Can you work these out from the model? Positions are in its coordinate system, mm. A direction names the side the tool comes from. Coordinates: 2 decimals unless noted, no trailing zeros. Order: outer loops, then holes, each group sorted by start corner. A loop starts at its lowest first (then second) coordinate and runs counter-clockwise, first axis right, second up. Notation, with made-up numbers: (-9, 83) - (-4, 83) arc R10 cw to (-4, 90) - close; hole circle Ø6 at (15.25, 35.5). An arc over 180 degrees is marked (long way). Return JSON: item names as keys, results as strings. Group by question number.
1) If I drill on line 1 along Z through (x, y) = (-95, 39.5); line 2 along X through (y, z) = (69.5, 89); line 3 along X through (y, z) = (42, 19), over which ranges is the centre line in solid material (lowest first)?
2) Imagine slicing it at B-B (x = -91.5). Write out the boundary of the cut face in (y, z).
3) Imagine slicing it at D-D (z = 70). Write out the boundary of the cut face in (x, y), and give its area (3 significant figures).
4) Imagine slicing it at C-C (y = 32). Write out the boundary of the cut face in (x, z), and give its area (3 significant figures).
5) Imagine slicing it at A-A (y = 64). Write out the boundary of the cut face in (x, z).
6) If we mould it in two halves opening along Z, with no side actions, what happens to faces 6 (the face through (-76, 11, 105.259)), 7 (the face through (38.401, 31, 52)), 8 (the face through (-75, 72, 68.159))? For each: pulls with the +Z half, pulls with the -Z half, needs draft (parallel to the pull), parting line crosses it, or undercut.
7) Which directions (+Z, -Z, +X, -X, +Y, -Y) give clear straight access to the entire face, cutting with the end or side of a thin tool? Please do faces 1 (the face through (-38, 82.151, 52)), 2 (the face through (-111.599, 31, 52)), 3 (the face through (-42.439, 11, 93)), 4 (the face through (-75, 77.151, 73)), 5 (the face through (-38, 32, 79.502)).
8) For pin 1 Ø2 at (x, y) = (-86, 36.5) entering from +Z; pin 2 Ø7 at (x, z) = (-90, 74) entering from -Y; pin 3 Ø1.5 at (x, y) = (13, 69.5) entering from +Z, each with a flat end and sliding along its axis, tell me the tip position at first contact or that it passes through.
```python
from build123d import *

# Parameters (mm, degrees)
F0_W      = 150
F0_H      = 100
F1_DEPTH  = 5
F2_W      = 5
F2_H      = 100
F3_DEPTH  = 100
F4_W      = 145
F4_H      = 5
F5_DEPTH  = 100
F6_W      = 5
F6_H      = 95
F7_DEPTH  = 100
F8_W      = 140
F8_H      = 5
F9_DEPTH  = 100
F10_W     = 140
F10_H     = 5
F11_DEPTH = 36.8
F12_W     = 10.8797177672
F12_H     = 90
F13_DEPTH = 36.8
F15_W     = 64.1449913383
F15_H     = 8.8397674263
F16_DEPTH = 36.8
F17_W     = 9.7464099526
F17_H     = 48.5053984448
F18_DEPTH = 37.1
F19_DEPTH = 1
F20_W     = 139.6295134723
F20_H     = 18.2434022427
F21_DEPTH = 85
F22_W     = 95
F22_H     = 2.5124400854
F23_DEPTH = 142.2
F25_DEPTH = 3


with BuildPart() as f1:
    # F0 (on Top) → F1 (new body)
    with BuildSketch(Plane.XY):
        with Locations((-36.598560214, 32.1514412761)):
            Rectangle(F0_W, F0_H)
    extrude(amount=F1_DEPTH)

    # F2 (on face) → F3 (join)
    with BuildSketch(Plane.XY.offset(5)):
        with Locations((-109.098560214, 32.1514412761)):
            Rectangle(F2_W, F2_H)
    extrude(amount=F3_DEPTH)

    # F4 (on face) → F5 (join)
    with BuildSketch(Plane.XY.offset(5)):
        with Locations((-34.098560214, 79.6514412761)):
            Rectangle(F4_W, F4_H)
    extrude(amount=F5_DEPTH)

    # F6 (on face) → F7 (join)
    with BuildSketch(Plane.XY.offset(5)):
        with Locations((35.901439786, 29.6514412761)):
            Rectangle(F6_W, F6_H)
    extrude(amount=F7_DEPTH)

    # F8 (on face) → F9 (join)
    with BuildSketch(Plane.XZ.offset(17.8485587239)):
        with Locations((-36.598560214, 65.6586462259)):
            Rectangle(F8_W, F8_H)
    extrude(amount=-F9_DEPTH)

    # F10 (on face) → F11 (join)
    with BuildSketch(Plane.XY.offset(68.1586462259)):
        with Locations((-36.598560214, -15.3485587239)):
            Rectangle(F10_W, F10_H)
    extrude(amount=F11_DEPTH)

    # F12 (on face) → F13 (join)
    with BuildSketch(Plane.XY.offset(68.1586462259)):
        with Locations((-36.9987897575, 32.1514412761)):
            Rectangle(F12_W, F12_H)
    extrude(amount=F13_DEPTH)

    # F15 (on face) → F16 (join)
    with BuildSketch(Plane.XY.offset(68.1586462259)):
        with Locations((-74.5111443102, 40.5214224011)):
            Rectangle(F15_W, F15_H)
    extrude(amount=F16_DEPTH)

    # F17 (on face) → F18 (join)
    with BuildSketch(Plane.XY.offset(68.1586462259)):
        with Locations((-75.8711062372, 11.1688547768)):
            Rectangle(F17_W, F17_H)
    extrude(amount=F18_DEPTH)

    # F19 (add): a face of the model
    f19_faces = [f1.faces().sort_by_distance(p)[0] for p in [
        (-75.8711062372, 35.4215539992, 86.7086462259),
    ]]
    extrude(f19_faces, amount=F19_DEPTH)

    # F20 (on face) → F21 (cut)
    with BuildSketch(Plane.XZ.offset(17.8485587239)):
        with Locations((-36.7838034779, 72.2803473473)):
            Rectangle(F20_W, F20_H)
    extrude(amount=-F21_DEPTH, mode=Mode.SUBTRACT)

    # F22 (on face) → F23 (join)
    with BuildSketch(Plane.YZ.offset(-106.598560214)):
        with Locations((29.6514412761, 78.2460346818)):
            Rectangle(F22_W, F22_H)
    extrude(amount=F23_DEPTH)

    # F24 (on face) → F25 (join)
    with BuildSketch(Plane(origin=(0, 0, 81.4020484686), x_dir=(1, 0, 0), z_dir=(0, 0, -1))):
        Polygon((33.0309532583, 17.8485587239), (-106.598560214, 17.8485587239), (-106.598560214, 12.8485587239), (-80.7443112135, 12.8485587239), (-70.9979012609, 12.8485587239), (-42.4386486411, 12.8485587239), (-31.5589308739, 12.8485587239), (33.0309532583, 12.8485587239), align=None)
    extrude(amount=F25_DEPTH)


solid = f1.part
```
Calculated:
{
 "1": {"line 1": "0 to 5, 76.99 to 79.5, 81.4 to 104.96", "line 2": "-111.6 to -106.6, -42.44 to -31.56, 33.4 to 38.4", "line 3": "-111.6 to -106.6, 33.4 to 38.4"},
 "2": {"outline": "(-17.85, 0) - (82.15, 0) - (82.15, 105) - (77.15, 105) - (77.15, 79.5) - (-12.85, 79.5) - (-12.85, 104.96) - (-17.85, 104.96) - (-17.85, 76.99) - (77.15, 76.99) - (77.15, 68.16) - (67.15, 68.16) - (67.15, 63.16) - (77.15, 63.16) - (77.15, 5) - (-17.85, 5) - close; (36.1, 81.4) - (44.94, 81.4) - (44.94, 104.96) - (36.1, 104.96) - close"},
 "3": {"outline": "(-111.6, -17.85) - (-106.6, -17.85) - (-106.6, 77.15) - (-42.44, 77.15) - (-42.44, 67.15) - (-31.56, 67.15) - (-31.56, 77.15) - (33.4, 77.15) - (33.4, -12.85) - (33.03, -12.85) - (33.03, -17.85) - (38.4, -17.85) - (38.4, 82.15) - (-111.6, 82.15) - close", "area": "1,810 mm2"},
 "4": {"outline": "(-111.6, 0) - (38.4, 0) - (38.4, 105) - (33.4, 105) - (33.4, 79.5) - (-106.6, 79.5) - (-106.6, 105) - (-111.6, 105) - close; (-80.74, 81.4) - (-71, 81.4) - (-71, 105.26) - (-80.74, 105.26) - close; (-42.44, 81.4) - (-31.56, 81.4) - (-31.56, 104.96) - (-42.44, 104.96) - close; hole (-106.6, 5) - (33.4, 5) - (33.4, 63.16) - (33.03, 63.16) - (33.03, 68.16) - (33.4, 68.16) - (33.4, 76.99) - (-106.6, 76.99) - close", "area": "2,590 mm2"},
 "5": {"outline": "(-111.6, 0) - (38.4, 0) - (38.4, 105) - (33.4, 105) - (33.4, 79.5) - (-106.6, 79.5) - (-106.6, 105) - (-111.6, 105) - close; (-42.44, 81.4) - (-31.56, 81.4) - (-31.56, 104.96) - (-42.44, 104.96) - close; hole (-106.6, 5) - (33.4, 5) - (33.4, 63.16) - (33.03, 63.16) - (33.03, 68.16) - (33.4, 68.16) - (33.4, 76.99) - (-106.6, 76.99) - close"},
 "6": {"face 6": "pulls with the +Z half", "face 7": "needs draft", "face 8": "undercut"},
 "7": {"face 1": "+Z, -Z, +X, -X, +Y", "face 2": "+Z, -Z, -X, +Y, -Y", "face 3": "+Z", "face 4": "-Y", "face 5": "none"},
 "8": {"pin 1": "z = 104.96", "pin 2": "y = -17.85", "pin 3": "z = 79.5"}
}
